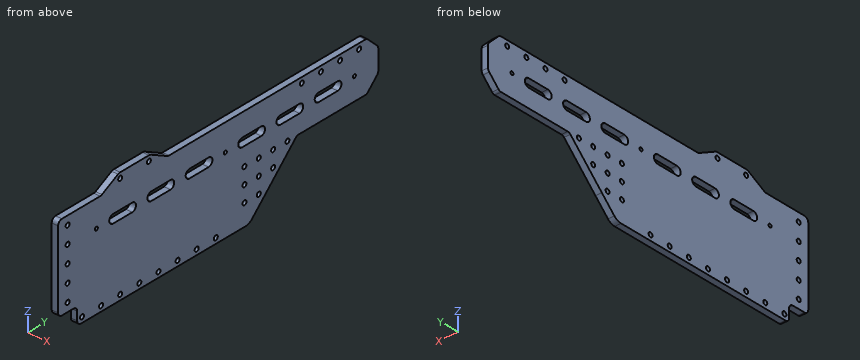
from build123d import *

# Parameters (mm, degrees)
SKETCH_1_W          = 80
SKETCH_1_H          = 315
SKETCH_1_R          = 1.6
SKETCH_1_H_2        = 20
SKETCH_1_R_2        = 2.1
EXTRUDE_1_DEPTH     = 6
SKETCH_2_W          = 16
SKETCH_2_H          = 180
EXTRUDE_2_DEPTH     = 6
SKETCH_3_W          = 34
SKETCH_3_H          = 85
CUT_EXTRUDE_1_DEPTH = 337.756588651
CHAMFER_1_SIZE      = 16
CHAMFER_2_SIZE      = 34
SKETCH_5_R          = 2.1
CUT_EXTRUDE_2_DEPTH = 337.756588651
SKETCH_5_3_R        = 2.1
EXTRUDE_3_DEPTH     = 6
SKETCH_6_R          = 2.1
CUT_EXTRUDE_3_DEPTH = 337.756588651
FILLET_START        = -1
FILLET_1_DEPTH      = 8
CHAMFER_3_SIZE      = 12
FILLET_2_DEPTH      = 8
FILLET_2_2_DEPTH    = 6
SKETCH_7_R          = 2.1
CUT_EXTRUDE_4_DEPTH = 337.756588651
CUT_EXTRUDE_5_DEPTH = 337.756588651


with BuildPart() as part:
    # 草图1 → 凸台-拉伸1 (new body)
    # profile 1 of 2: a face of its own
    with BuildSketch(Plane(origin=(0, 0, 0), x_dir=(0, 0, -1), z_dir=(1, 0, 0))):
        with Locations((32, 167.5)):
            Rectangle(SKETCH_1_W, SKETCH_1_H)
        with Locations((17, 300)):
            Circle(SKETCH_1_R, mode=Mode.SUBTRACT)
        with Locations((17, 165)):
            Circle(SKETCH_1_R, mode=Mode.SUBTRACT)
        with Locations((17, 30)):
            Circle(SKETCH_1_R, mode=Mode.SUBTRACT)
    # profile 2 of 2: a face of its own
    with BuildSketch(Plane(origin=(0, 0, 0), x_dir=(0, 0, -1), z_dir=(1, 0, 0))):
        with Locations((32, 0)):
            Rectangle(SKETCH_1_W, SKETCH_1_H_2)
        with Locations((64, 0)):
            Circle(SKETCH_1_R_2, mode=Mode.SUBTRACT)
        with Locations((48, 0)):
            Circle(SKETCH_1_R_2, mode=Mode.SUBTRACT)
        with Locations((32, 0)):
            Circle(SKETCH_1_R_2, mode=Mode.SUBTRACT)
        with Locations((16, 0)):
            Circle(SKETCH_1_R_2, mode=Mode.SUBTRACT)
        Circle(SKETCH_1_R_2, mode=Mode.SUBTRACT)
    extrude(amount=EXTRUDE_1_DEPTH)

    # 草图2 → 凸台-拉伸2 (add)
    with BuildSketch(Plane.ZY):
        with Locations((-80, 100)):
            Rectangle(SKETCH_2_W, SKETCH_2_H)
    extrude(amount=-EXTRUDE_2_DEPTH)

    # 草图3 → 切除-拉伸1 (cut, through all)
    with BuildSketch(Plane.ZY):
        with Locations((-55, 282.5)):
            Rectangle(SKETCH_3_W, SKETCH_3_H)
    extrude(amount=-CUT_EXTRUDE_1_DEPTH, mode=Mode.SUBTRACT)

    # 倒角1
    chamfer_1_edges = [part.edges().sort_by_distance(p)[0] for p in [
        (3, 190, -72),
    ]]
    chamfer(chamfer_1_edges, length=CHAMFER_1_SIZE - 0.0001)  # a hair under: the kernel refuses the full size

    # 倒角2
    chamfer_2_edges = [part.edges().sort_by_distance(p)[0] for p in [
        (3, 240, -72),
    ]]
    chamfer(chamfer_2_edges, length=CHAMFER_2_SIZE - 0.0001)  # a hair under: the kernel refuses the full size

    # 草图5 → 切除-拉伸2 (cut, through all)
    with BuildSketch(Plane.ZY):
        with Locations((-83, 15)):
            Circle(SKETCH_5_R)
        with Locations((-83, 35)):
            Circle(SKETCH_5_R)
        with Locations((-83, 55)):
            Circle(SKETCH_5_R)
        with Locations((-83, 75)):
            Circle(SKETCH_5_R)
        with Locations((-83, 95)):
            Circle(SKETCH_5_R)
        with Locations((-83, 115)):
            Circle(SKETCH_5_R)
        with Locations((-83, 135)):
            Circle(SKETCH_5_R)
        with Locations((-83, 155)):
            Circle(SKETCH_5_R)
    extrude(amount=-CUT_EXTRUDE_2_DEPTH, mode=Mode.SUBTRACT)

    # 草图5<3> → 凸台-拉伸3 (add)
    with BuildSketch(Plane.ZY):
        with BuildLine():
            ThreePointArc((17.411764706, 52.647058824), (17.850712501, 53.787321875), (18, 55))
            Line((18, 55), (18, 85))
            ThreePointArc((18, 85), (17.850712501, 86.212678125), (17.411764706, 87.352941176))
            Line((17.411764706, 87.352941176), (8, 105))
            Line((8, 105), (8, 35))
            Line((8, 35), (17.411764706, 52.647058824))
        make_face()
        with Locations((13, 85)):
            Circle(SKETCH_5_3_R, mode=Mode.SUBTRACT)
        with Locations((13, 55)):
            Circle(SKETCH_5_3_R, mode=Mode.SUBTRACT)
    extrude(amount=-EXTRUDE_3_DEPTH)

    # 草图6 → 切除-拉伸3 (cut, through all)
    with BuildSketch(Plane.ZY):
        with Locations((-68, 185)):
            Circle(SKETCH_6_R)
        with Locations((-53, 185)):
            Circle(SKETCH_6_R)
        with Locations((-38, 185)):
            Circle(SKETCH_6_R)
        with Locations((-68, 200)):
            Circle(SKETCH_6_R)
        with Locations((-53, 200)):
            Circle(SKETCH_6_R)
        with Locations((-38, 200)):
            Circle(SKETCH_6_R)
        with Locations((-68, 215)):
            Circle(SKETCH_6_R)
        with Locations((-53, 215)):
            Circle(SKETCH_6_R)
        with Locations((-38, 215)):
            Circle(SKETCH_6_R)
        with Locations((-68, 230)):
            Circle(SKETCH_6_R)
        with Locations((-53, 230)):
            Circle(SKETCH_6_R)
        with Locations((-38, 230)):
            Circle(SKETCH_6_R)
        with Locations((-83, 200)):
            Circle(SKETCH_6_R)
        with Locations((-83, 215)):
            Circle(SKETCH_6_R)
        with Locations((-83, 230)):
            Circle(SKETCH_6_R)
    extrude(amount=-CUT_EXTRUDE_3_DEPTH, mode=Mode.SUBTRACT)

    # 圆角1: read off the stored shape, not the designer's step
    # 圆角1 outline → 圆角1 (cut)
    with BuildSketch(Plane.YZ.offset(FILLET_START)):
        with BuildLine():
            ThreePointArc((192.928932188, -85.071067812), (189.6846987, -87.238795325), (185.857864376, -88))
            Line((185.857864376, -88), (190, -88))
            Line((190, -88), (192.928932188, -85.071067812))
        make_face()
    extrude(amount=FILLET_1_DEPTH, mode=Mode.SUBTRACT)

    # 倒角3
    chamfer_3_edges = [part.edges().sort_by_distance(p)[0] for p in [
        (3, 325, 8),
        (3, 325, -38),
    ]]
    chamfer(chamfer_3_edges, length=CHAMFER_3_SIZE)

    # 圆角2: read off the stored shape, not the designer's step
    # 圆角2 outline → 圆角2 (cut)
    with BuildSketch(Plane.YZ.offset(FILLET_START)):
        with BuildLine():
            Line((313, -38), (314.171572875, -36.828427125))
            ThreePointArc((314.171572875, -36.828427125), (312.87387948, -37.69551813), (311.343145751, -38))
            Line((311.343145751, -38), (313, -38))
        make_face()
        with BuildLine():
            ThreePointArc((311.343145751, 8), (312.87387948, 7.69551813), (314.171572875, 6.828427125))
            Line((314.171572875, 6.828427125), (313, 8))
            Line((313, 8), (311.343145751, 8))
        make_face()
        with BuildLine():
            ThreePointArc((323.828427125, -2.828427125), (324.69551813, -4.12612052), (325, -5.656854249))
            Line((325, -5.656854249), (325, -4))
            Line((325, -4), (323.828427125, -2.828427125))
        make_face()
        with BuildLine():
            ThreePointArc((325, -24.343145751), (324.69551813, -25.87387948), (323.828427125, -27.171572875))
            Line((323.828427125, -27.171572875), (325, -26))
            Line((325, -26), (325, -24.343145751))
        make_face()
        with BuildLine():
            Line((10, -88), (14, -88))
            ThreePointArc((14, -88), (11.171572875, -86.828427125), (10, -84))
            Line((10, -84), (10, -88))
        make_face()
        with BuildLine():
            Line((-10, 8), (-10, 4))
            ThreePointArc((-10, 4), (-8.828427125, 6.828427125), (-6, 8))
            Line((-6, 8), (-10, 8))
        make_face()
        with BuildLine():
            Line((-10, -72), (-6, -72))
            ThreePointArc((-6, -72), (-8.828427125, -70.828427125), (-10, -68))
            Line((-10, -68), (-10, -72))
        make_face()
    extrude(amount=FILLET_2_DEPTH, mode=Mode.SUBTRACT)

    # Fillet 2 2 outline → Fillet 2 2 (add)
    with BuildSketch(Plane.YZ):
        with BuildLine():
            ThreePointArc((238.828427125, -39.171572875), (240.12612052, -38.30448187), (241.656854249, -38))
            Line((241.656854249, -38), (240, -38))
            Line((240, -38), (238.828427125, -39.171572875))
        make_face()
        with BuildLine():
            Line((105, 8), (106, 8))
            ThreePointArc((106, 8), (105.0298575, 8.119429999), (104.117647059, 8.470588235))
            Line((104.117647059, 8.470588235), (105, 8))
        make_face()
        with BuildLine():
            ThreePointArc((35.882352941, 8.470588235), (34.9701425, 8.119429999), (34, 8))
            Line((34, 8), (35, 8))
            Line((35, 8), (35.882352941, 8.470588235))
        make_face()
        with BuildLine():
            ThreePointArc((6, -72), (8.828427125, -73.171572875), (10, -76))
            Line((10, -76), (10, -72))
            Line((10, -72), (6, -72))
        make_face()
    extrude(amount=FILLET_2_2_DEPTH)

    # 草图7 → 切除-拉伸4 (cut, through all)
    with BuildSketch(Plane.ZY):
        with Locations((3, 305)):
            Circle(SKETCH_7_R)
        with Locations((3, 285)):
            Circle(SKETCH_7_R)
        with Locations((3, 265)):
            Circle(SKETCH_7_R)
        with Locations((3, 245)):
            Circle(SKETCH_7_R)
    extrude(amount=-CUT_EXTRUDE_4_DEPTH, mode=Mode.SUBTRACT)

    # 草图8 → 切除-拉伸5 (cut, through all)
    with BuildSketch(Plane.ZY):
        with BuildLine():
            Line((-21, 222.5), (-21, 242.5))
            ThreePointArc((-21, 242.5), (-17, 246.5), (-13, 242.5))
            Line((-13, 242.5), (-13, 222.5))
            ThreePointArc((-13, 222.5), (-17, 218.5), (-21, 222.5))
        make_face()
        with BuildLine():
            Line((-21, 262.5), (-21, 282.5))
            ThreePointArc((-21, 282.5), (-17, 286.5), (-13, 282.5))
            Line((-13, 282.5), (-13, 262.5))
            ThreePointArc((-13, 262.5), (-17, 258.5), (-21, 262.5))
        make_face()
        with BuildLine():
            Line((-13, 182.5), (-13, 202.5))
            ThreePointArc((-13, 202.5), (-17, 206.5), (-21, 202.5))
            Line((-21, 202.5), (-21, 182.5))
            ThreePointArc((-21, 182.5), (-17, 178.5), (-13, 182.5))
        make_face()
        with BuildLine():
            Line((-21, 147.5), (-21, 127.5))
            ThreePointArc((-21, 127.5), (-17, 123.5), (-13, 127.5))
            Line((-13, 127.5), (-13, 147.5))
            ThreePointArc((-13, 147.5), (-17, 151.5), (-21, 147.5))
        make_face()
        with BuildLine():
            Line((-21, 107.5), (-21, 87.5))
            ThreePointArc((-21, 87.5), (-17, 83.5), (-13, 87.5))
            Line((-13, 87.5), (-13, 107.5))
            ThreePointArc((-13, 107.5), (-17, 111.5), (-21, 107.5))
        make_face()
        with BuildLine():
            Line((-21, 67.5), (-21, 47.5))
            ThreePointArc((-21, 47.5), (-17, 43.5), (-13, 47.5))
            Line((-13, 47.5), (-13, 67.5))
            ThreePointArc((-13, 67.5), (-17, 71.5), (-21, 67.5))
        make_face()
    extrude(amount=-CUT_EXTRUDE_5_DEPTH, mode=Mode.SUBTRACT)


solid = part.part
Source: CAD feature listing. Evaluate the final solid. Frame: model axes, mm. Give positions to 0.01 mm unless a question says otherwise; leave off trailing zeros. Write each loop counter-clockwise with the first axis right and the second up, starting at its lowest first coordinate (ties: lowest second). Pieces come first, ordered by that corner, then holes. Notation, with made-up numbers: M 67.25,-19 L 80.25,-19 A22 ccw 80.25,11 Z; hole C 87,-27 d8. An arc over 180 degrees is marked long. Answer as a JSON object with one key per item and string values.
Q1. Ray query, line 1 along Z through (x, y) = (4, 272); line 2 along Z through (x, y) = (5.25, 184.5); line 3 along Y through (x, z) = (1.4, -53). Return the intervals inside material, ascending.
Geometry check:
{"line 1": "z = -38 to -21, -13 to 8", "line 2": "z = -88 to -70.04, -65.96 to -55.04, -50.96 to -40.04, -35.96 to -21, -13 to 8", "line 3": "y = -10 to 182.9, 187.1 to 197.9, 202.1 to 212.9, 217.1 to 225"}
Q2. Cut plane A-A, the plane y = 141. Return the cut outline in (x, z), then the cut area to 3 significant figures.
Geometry check:
{"outline": "M 0,-88 L 6,-88 L 6,-21 L 0,-21 Z; M 0,-13 L 6,-13 L 6,8 L 0,8 Z", "area": "528 mm^2"}
Q3. Cut plane C-C, the plane y = 23. Return the cut outline in (x, z), then the cut area to 3 significant figures.
Geometry check:
{"outline": "M 0,-88 L 6,-88 L 6,8 L 0,8 Z", "area": "576 mm^2"}
Q4. Cut plane B-B, the plane x = 1.25. Count the separate pieces of the cut face and the enclosed holes in it, then the cut area to 3 significant figures.
Geometry check:
{"separate pieces": "1", "enclosed holes": "37", "area": "25,000 mm^2"}
Q5. Contact query for flat-ended pins moving along their axis: P1, Ø2, axis at x = 1.5, z = -77, coming from the +Y side; P2, Ø3, axis at x = 2, z = -46.5, coming from the +Y side; P3, Ø3, axis at y = 30, z = -17, coming from the +X side. Output: stop coordinate, or through.
Geometry check:
{"P1": "stops at y = 202", "P2": "stops at y = 233", "P3": "passes through"}
